from build123d import *

# Parameters (mm, degrees)
SKETCH2_R           = 20
SKETCH4_R           = 20
BOSS_EXTRUDE1_DEPTH = 33.2


with BuildPart() as part:
    # Sweep1: sweep along a path in Sketch1
    with BuildLine(Plane.XY) as sweep1_path:
        Line((0, 0), (75, 0))
    # Sketch2 → Sweep1 (sweep)
    with BuildSketch(Plane(origin=(0, 0, 0), x_dir=(0, 0, -1), z_dir=(1, 0, 0))):
        Circle(SKETCH2_R)
    sweep(path=sweep1_path.line)

    # Sketch4 → Boss-Extrude1 (add)
    with BuildSketch(Plane(origin=(0, 0, 0), x_dir=(1, 0, 0), z_dir=(0, 1, 0))):
        with Locations(Location((45, 0, 0), (0, 0, 270))):
            Circle(SKETCH4_R)
    extrude(amount=-BOSS_EXTRUDE1_DEPTH)

    # Sketch5 → Revolve1 (revolve)
    with BuildSketch(Plane(origin=(0, 0, 0), x_dir=(1, 0, 0), z_dir=(0, 1, 0))):
        Polygon((0, 0), (-110, 0), (-110, 7), (-80, 7), (-80, 15), (0, 15), align=None)
    revolve(axis=Axis((-110, 0, 0), (-1, 0, 0)))


solid = part.part
Input: part model. Units: mm. Frame: model coordinates. A direction names the side the tool comes from. Coordinates: 2 decimals unless noted, no trailing zeros. Order: outer loops, then holes, each group sorted by start corner. A loop starts at its lowest first (then second) coordinate and runs counter-clockwise, first axis right, second up. Notation, with made-up numbers: M 3,-6.75 L 26,-6.75 A7 cw 26,-0.75 Z; hole C 78.5,-37 d11. An arc over 180 degrees is marked long. Answer as CSV lines item,"result".
1. Access query for faces 1 (the cylindrical face through (33, -20, -16)), 2 (the flat face through (75, 0, 0)), 3 (the cylindrical face through (-39.44, -0.66, 14.985)). Directions: +Z, -Z, +X, -X, +Y, -Y. A direction counts if a zero-diameter tool reaches every point of the face in a straight line with its end or side. Return the directions, or none.
Reported:
face 1,"-Y"
face 2,"+Z, -Z, +X, +Y, -Y"
face 3,"-X"
2. Section B-B (x = 45). Return the cut outline in (y, z).
Reported:
outline,"M -33.2,-20 L 0,-20 A20 ccw 0,20 L -33.2,20 Z"
3. First-contact query: P1, Ø1, axis at x = 19, y = -2.5, coming from the -Z side; P2, Ø2, axis at y = -20, z = 7.5, coming from the +X side; P3, Ø2, axis at x = -87, y = -2.5, coming from the -Z side. Flat tips, straight axial feed; report the tip coordinate or a pass-through.
Reported:
P1,"z = -19.9"
P2,"x = 63.91"
P3,"z = -6.84"
4. Section D-D (z = -9). Return the cut outline in (x, y).
Reported:
outline,"M -80,-12 L 0,-12 L 0,-17.86 L 27.14,-17.86 L 27.14,-33.2 L 62.86,-33.2 L 62.86,-17.86 L 75,-17.86 L 75,17.86 L 0,17.86 L 0,12 L -80,12 Z"
5. Material intervals for line 1 (X direction, y = -7, z = 17); line 2 (X direction, y = 4, z = -8); line 3 (Z direction, x = 23, y = -11.5), sorted ascending. Write a range as from..to.
Reported:
line 1,"0..75"
line 2,"-80..75"
line 3,"-16.36..16.36"
6. Section A-A (z = 0). Return the cut outline in (x, y), then the cut area to 3 significant figures.
Reported:
outline,"M -110,-7 L -80,-7 L -80,-15 L 0,-15 L 0,-20 L 25,-20 L 25,-33.2 L 65,-33.2 L 65,-20 L 75,-20 L 75,20 L 0,20 L 0,15 L -80,15 L -80,7 L -110,7 Z"
area,"6,350 mm2"
7. Section C-C (y = -24). Return the cut outline in (x, z).
Reported:
outline,"C 45,0 d40"
